Geometry: final body of the model. Coordinates: model frame, mm. Face numbers are marked on the shaded views. A direction names the side the tool comes from. Give positions to 0.01 mm unless a question says otherwise; leave off trailing zeros. Write each loop counter-clockwise with the first axis right and the second up, starting at its lowest first coordinate (ties: lowest second). Pieces come first, ordered by that corner, then holes.
Q1. Pin query (flat end, axial travel): pin 1 Ø2 at (x, y) = (30.5, -18.5) entering from -Z; pin 2 Ø2 at (x, z) = (21.5, 1) entering from -Y; pin 3 Ø5 at (y, z) = (0, -17.5) entering from -X. Return the tip coordinate at first contact, or that it passes through.
Q2. Reachability of the marked faces 1, 2 and 3 from +Z, -Z, +X, -X, +Y, -Y: full face, straight path, thin tool, end or side. Return the list, or none.
Q3. Section C-C (z = 0). State how many separate pieces and enclosed holes the cut face has, plus the area to 3 significant figures.
Q4. Section B-B (z = -31.5). Return the cut outline in (x, y).
Q5. Section D-D (x = 12). Return the cut outline in (y, z), plus the area to 3 significant figures.
Q6. Line query: line 1 (Z direction, x = 36.8, y = 0); line 2 (Z direction, x = 21, y = 0.5) (3 decimals); line 3 (Y direction, x = 17, z = 11). Output: solid intervals per line, ascending.
Q7. Section A-A (y = -32). Return the cut outline in (x, z), plus the area to 3 significant figures.
Q8. Mould query, pull axis Y, two halves, no side actions, for the marked faces 4, 5 and 6. Classes: +Y half, -Y half, draft (parallel to the pull), parting line (faces both ways), or undercut.
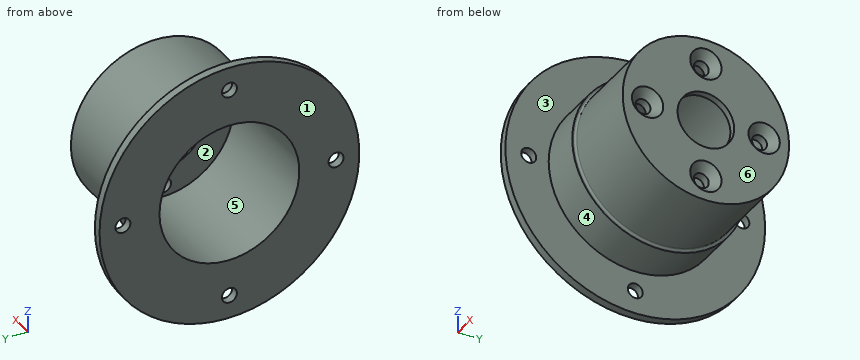
from build123d import *

# Parameters (mm, degrees)
CSK_FOR_M4_FLAT_HEAD_MACHINE_SCREW1_D           = 4.5
CSK_FOR_M4_FLAT_HEAD_MACHINE_SCREW1_DEPTH       = 5
CSK_FOR_M4_FLAT_HEAD_MACHINE_SCREW1_CSINK_D     = 9.4
CSK_FOR_M4_FLAT_HEAD_MACHINE_SCREW1_CSINK_ANGLE = 90
FILLET1_R                                       = 0.6
M4_CLEARANCE_HOLE1_D                            = 4.5
M4_CLEARANCE_HOLE1_DEPTH                        = 2.5


with BuildPart() as part:
    # Sketch2 → Revolve1 (revolve)
    with BuildSketch(Plane.XY):
        Polygon((0, 21), (35, 21), (35, 12.5), (38, 12.5), (38, 8.5), (40, 8.5), (40, 25), (15, 25), (15, 26), (2.5, 26), (2.5, 39), (0, 39), (0, 26), align=None)
    revolve(axis=Axis((-64.103352454, 0, 0), (1, 0, 0)))

    # CSK for M4 Flat Head Machine Screw1
    with Locations(Plane(origin=(40, 0, 0), x_dir=(0, 0, -1), z_dir=(1, 0, 0))):
        with Locations((0, 17.5), (17.5, 0), (0, -17.5), (-17.5, 0)):
            CounterSinkHole(CSK_FOR_M4_FLAT_HEAD_MACHINE_SCREW1_D / 2, CSK_FOR_M4_FLAT_HEAD_MACHINE_SCREW1_CSINK_D / 2, depth=CSK_FOR_M4_FLAT_HEAD_MACHINE_SCREW1_DEPTH, counter_sink_angle=CSK_FOR_M4_FLAT_HEAD_MACHINE_SCREW1_CSINK_ANGLE)

    # Fillet1
    fillet1_edges = [part.edges().sort_by_distance(p)[0] for p in [
        (15, -25, 0),
    ]]
    fillet(fillet1_edges, radius=FILLET1_R)

    # M4 Clearance Hole1
    with Locations(Plane.ZY):
        with Locations((0, 32), (0, -32), (32, 0), (-32, 0)):
            Hole(M4_CLEARANCE_HOLE1_D / 2, depth=M4_CLEARANCE_HOLE1_DEPTH)


solid = part.part
Computed:
1. pin 1: stops at z = -17.85
1. pin 2: stops at y = -25
1. pin 3: stops at x = 35
2. face 1: +Z, -Z, -X, +Y, -Y
2. face 2: -X
2. face 3: +X
3. separate pieces: 6
3. enclosed holes: 0
3. area: 437 mm2
4. outline: (0, -22.99) - (2.5, -22.99) - (2.5, -2.19) - (0, -2.19) - close; (0, 2.19) - (2.5, 2.19) - (2.5, 22.99) - (0, 22.99) - close
5. outline: circle Ø52 at (0, 0); hole circle Ø42 at (0, 0)
5. area: 738 mm2
6. line 1: z = -25 to -19.75, -15.25 to -12.5, 12.5 to 15.25, 19.75 to 25
6. line 2: z = -24.995 to -20.994, 20.994 to 24.995
6. line 3: y = -22.45 to -17.89, 17.89 to 22.45
7. outline: (0, -22.29) - (2.5, -22.29) - (2.5, -2.25) - (0, -2.25) - close; (0, 2.25) - (2.5, 2.25) - (2.5, 22.29) - (0, 22.29) - close
7. area: 100 mm2
8. face 4: parting line
8. face 5: undercut
8. face 6: draft
